Design review of the part built by this model. Coordinates are the model's own, in mm. A direction names the side the tool comes from. Coordinates: 2 decimals unless noted, no trailing zeros. Loops run counter-clockwise (first coordinate to the right, second up) from the corner with the lowest first, then second, coordinate; pieces in that order, holes last. Notation, with made-up numbers: (1, 42.25) -> (30, 42.25) arc R10 ccw to (30, 60.25) -> close; hole circle Ø10 at (85, 5.25). An arc over 180 degrees is marked (long way). One line per item, written item: value. Start each with the question number.
1. For probe 1 along Z at (x, y) = (13.5, 10.5); probe 2 along Z at (x, y) = (-53, 19.5); probe 3 along X at (y, z) = (11, 2.2), list the stretches that pass through material, from the lowest coordinate up.
2. Add section C-C on x = -18. Write out the cut boundary in (y, z).
3. Draft analysis for pull direction Y (two halves, no side actions). For faces 1 (the flat face through (-1.547, 14.682, 1.493)), 2 (the flat face through (-37.66, 48.03, 1.49)), 3 (the cylindrical face through (-37.505, -10.165, 2.43)), state which applies: pulls with the +Y half, pulls with the -Y half, needs draft (parallel to the pull), parting line crosses it, or undercut.
4. Machinability: for faces 4 (the flat face through (-50.7, -8.1, 1.5)), 5 (the flat face through (-24.15, -13.37, 1.49)), 6 (the flat face through (-31.355, 46.756, 1.493)), 7 (the flat face through (-21, 42, 2)), 8 (the cylindrical face through (-12.11, 34.55, 2.49)), which of the approach directions +Z, -Z, +X, -X, +Y, -Y give a long, thin tool a straight path to every point of the face, cutting with its end or side? Answer none if there is none.
5. Add section A-A on x = -30. Write out the cut boundary in (y, z), plus the area to 3 significant figures.
6. Insertion check: pin 1 (1.5 mm diameter, centred on x = -35.5, z = 1, fed in from +Y); pin 2 (3 mm diameter, centred on y = 32.5, z = 1.5, fed in from +X); pin 3 (3 mm diameter, centred on x = -47.5, z = 3, fed in from +Y). Each pin has a flat end and moves straight along its axis. Give the tip position at first contact, or say it passes through.
7. Add section D-D on y = -25. Write out the cut boundary in (x, z), plus the area to 3 significant figures.
8. Add section B-B on y = 4. Write out the cut boundary in (x, z).
```python
from build123d import *

# Parameters (mm, degrees)
F0_R     = 9.34954834
F1_DEPTH = 2
F2_R     = 9.9314109332
F3_DEPTH = 3
F4_R     = 24.7483511113
F4_R_2   = 9.9812356791
F5_DEPTH = 4
F6_R     = 21.0489130691
F6_R_2   = 7.6981825143
F7_DEPTH = 5
F8_R     = 50.7680243712
F8_R_2   = 10.127452023
F9_DEPTH = 1


with BuildPart() as f1:
    # F0 (on Top) → F1 (new body)
    with BuildSketch(Plane.XY):
        Polygon((-2.3253114279, 7.0025283952), (0.7141198772, 9.8394449822), (-3.8715197243, 19.6616453301), align=None)
        Polygon((-1.3632647613, -0.8739403047), (-2.3253114279, 7.0025283952), (-7.2580368413, 2.3984662733), (-8.5569428744, -4.2228637399), align=None)
        Polygon((-7.2580368413, 2.3984662733), (-2.3253114279, 7.0025283952), (-3.8715197243, 19.6616453301), align=None)
        Polygon((-7.2580368413, 2.3984662733), (-3.8715197243, 19.6616453301), (-11.3136030379, 35.6021988113), (-26.6853706311, 44.1575836885), (-44.1454681102, 42.0056437837), (-57.0322600669, 30.0299833677), (-60.3811104422, 12.7594578836), (-52.9738182843, -3.1972921683), (-37.5834241603, -11.7191240163), (-20.1186738854, -9.6052774824), align=None)
        with Locations((-32.1363285184, 16.2093285471)):
            Circle(F0_R, mode=Mode.SUBTRACT)
        Polygon((-5.4177280207, 32.3207622651), (-3.8715197243, 19.6616453301), (-1.7848262074, 30.2988169654), align=None)
        Polygon((-11.3136030379, 35.6021988113), (-3.8715197243, 19.6616453301), (-5.4177280207, 32.3207622651), align=None)
        Polygon((-8.5569428744, -4.2228637399), (-7.2580368413, 2.3984662733), (-20.1186738854, -9.6052774824), align=None)
        Polygon((-26.6853706311, 44.1575836885), (-11.3136030379, 35.6021988113), (-14.1680303391, 41.7162328976), align=None)
        Polygon((-14.1680303391, 41.7162328976), (-11.3136030379, 35.6021988113), (-5.4177280207, 32.3207622651), (-6.3797746873, 40.197230965), align=None)
        Polygon((-8.5569428744, -4.2228637399), (-20.1186738854, -9.6052774824), (-9.3572987281, -8.3027741418), align=None)
        Polygon((-31.6804048965, -14.9876912249), (-20.1186738854, -9.6052774824), (-37.5834241603, -11.7191240163), align=None)
        Polygon((-28.0431009638, -17.0017067365), (-20.1186738854, -9.6052774824), (-31.6804048965, -14.9876912249), align=None)
        Polygon((-26.6853706311, 44.1575836885), (-14.1680303391, 41.7162328976), (-15.9268624188, 45.4835592832), align=None)
        Polygon((-39.202710923, 46.5989344794), (-26.6853706311, 44.1575836885), (-36.1570982709, 49.4292139626), align=None)
        Polygon((-44.1454681102, 42.0056437837), (-26.6853706311, 44.1575836885), (-39.202710923, 46.5989344794), align=None)
        Polygon((-44.2820672543, -12.5298944689), (-37.5834241603, -11.7191240163), (-52.9738182843, -3.1972921683), align=None)
        Polygon((-31.6804048965, -14.9876912249), (-37.5834241603, -11.7191240163), (-44.2820672543, -12.5298944689), (-38.8740830096, -18.3366146601), align=None)
        Polygon((-57.0322600669, 30.0299833677), (-44.1454681102, 42.0056437837), (-50.8423266141, 41.1802625354), align=None)
        Polygon((-50.8423266141, 41.1802625354), (-44.1454681102, 42.0056437837), (-39.202710923, 46.5989344794), (-46.9909665748, 48.117936412), align=None)
        Polygon((-44.2820672543, -12.5298944689), (-52.9738182843, -3.1972921683), (-48.4096161882, -13.0294724686), align=None)
        Polygon((-61.6655693143, 6.1353101322), (-52.9738182843, -3.1972921683), (-60.3811104422, 12.7594578836), align=None)
        Polygon((-62.4570231615, 2.0536635052), (-52.9738182843, -3.1972921683), (-61.6655693143, 6.1353101322), align=None)
        Polygon((-57.0322600669, 30.0299833677), (-50.8423266141, 41.1802625354), (-54.968775925, 40.6716817015), align=None)
        Polygon((-63.2221935197, 18.8797042), (-57.0322600669, 30.0299833677), (-64.9728031974, 22.650858418), align=None)
        Polygon((-60.3811104422, 12.7594578836), (-57.0322600669, 30.0299833677), (-63.2221935197, 18.8797042), align=None)
        Polygon((-61.6655693143, 6.1353101322), (-60.3811104422, 12.7594578836), (-63.2221935197, 18.8797042), (-67.0735535589, 11.9420303234), align=None)
    extrude(amount=F1_DEPTH)

    # F2 (on Top) → F3 (join)
    with BuildSketch(Plane.XY):
        with BuildLine():
            ThreePointArc((-3.9161127061, 19.6736101061), (-12.2738953914, 34.7283526931), (-26.6918931156, 44.142127037))
            ThreePointArc((-26.6918931156, 44.142127037), (-44.0241929939, 41.7700167457), (-57.0044443011, 30.04190512))
            ThreePointArc((-57.0044443011, 30.04190512), (-61.0707346416, 12.665349743), (-52.9653914273, -3.2337950543))
            ThreePointArc((-52.9653914273, -3.2337950543), (-37.2668042058, -10.2120179587), (-20.0973842293, -9.6185086295))
            ThreePointArc((-20.0973842293, -9.6185086295), (-7.0292200811, 2.277912207), (-3.9161127061, 19.6736101061))
        make_face()
        with Locations((-31.4443483949, 17.2526501119)):
            Circle(F2_R, mode=Mode.SUBTRACT)
    extrude(amount=F3_DEPTH)

    # F4 (on Top) → F5 (join)
    with BuildSketch(Plane.XY):
        with Locations((-32.1926809847, 16.7406294495)):
            Circle(F4_R)
        with Locations((-32.1926809847, 16.7406294495)):
            Circle(F4_R_2, mode=Mode.SUBTRACT)
    extrude(amount=F5_DEPTH)

    # F6 (on Top) → F7 (join)
    with BuildSketch(Plane.XY):
        with Locations((-32.0071727037, 16.5551174432)):
            Circle(F6_R)
        with Locations((-32.0071727037, 16.5551174432)):
            Circle(F6_R_2, mode=Mode.SUBTRACT)
    extrude(amount=F7_DEPTH)

    # F8 (on Top) → F9 (join)
    with BuildSketch(Plane.XY):
        with Locations((-32.0829190314, 16.9553998858)):
            Circle(F8_R)
        with Locations((-32.0829190314, 16.9553998858)):
            Circle(F8_R_2, mode=Mode.SUBTRACT)
    extrude(amount=F9_DEPTH)


solid = f1.part
```
Worked answers:
1. probe 1: z = 0 to 1
1. probe 2: z = 0 to 4
1. probe 3: x = -60.81 to -37.34, -26.68 to -3.99
2. outline: (-31.82, 0) -> (65.73, 0) -> (65.73, 1) -> (45.23, 1) -> (45.23, 2) -> (39.7, 2) -> (39.7, 3) -> (37.01, 3) -> (37.01, 4) -> (32.27, 4) -> (32.27, 5) -> (0.84, 5) -> (0.84, 4) -> (-3.53, 4) -> (-3.53, 3) -> (-8.6, 3) -> (-8.6, 2) -> (-9.35, 2) -> (-9.35, 1) -> (-31.82, 1) -> close
3. face 1: undercut
3. face 2: pulls with the +Y half
3. face 3: pulls with the -Y half
4. face 4: +Z, -X, -Y
4. face 5: +Z, +X, -Y
4. face 6: +Z, +Y
4. face 7: +Z
4. face 8: +Z, +X, +Y
5. outline: (-33.77, 0) -> (9.12, 0) -> (9.12, 5) -> (-4.4, 5) -> (-4.4, 4) -> (-7.91, 4) -> (-7.91, 3) -> (-10.91, 3) -> (-10.91, 2) -> (-15.92, 2) -> (-15.92, 1) -> (-33.77, 1) -> close; (23.99, 0) -> (67.68, 0) -> (67.68, 1) -> (46, 1) -> (46, 2) -> (44.5, 2) -> (44.5, 3) -> (41.39, 3) -> (41.39, 4) -> (37.51, 4) -> (37.51, 5) -> (23.99, 5) -> close
5. area: 236 mm²
6. pin 1: stops at y = 67.65
6. pin 2: stops at x = 16.68
6. pin 3: stops at y = 48.12
7. outline: (-60.67, 0) -> (-3.5, 0) -> (-3.5, 1) -> (-60.67, 1) -> close
7. area: 57.2 mm²
8. outline: (-81.17, 0) -> (17, 0) -> (17, 1) -> (-1.96, 1) -> (-1.96, 2) -> (-6.16, 2) -> (-6.16, 3) -> (-10.98, 3) -> (-10.98, 4) -> (-15.11, 4) -> (-15.11, 5) -> (-48.9, 5) -> (-48.9, 4) -> (-53.41, 4) -> (-53.41, 3) -> (-58.43, 3) -> (-58.43, 2) -> (-62.08, 2) -> (-62.08, 1) -> (-81.17, 1) -> close
